Can you work these out from the model? Positions are in its coordinate system, mm. A direction names the side the tool comes from. Coordinates: 2 decimals unless noted, no trailing zeros. Loops run counter-clockwise (first coordinate to the right, second up) from the corner with the lowest first, then second, coordinate; pieces in that order, holes last. Notation, with made-up numbers: M 64.25,16 L 91.25,16 A33 ccw 91.25,49 Z; hole C 12.25,56.25 d9. An arc over 180 degrees is marked long. Answer as a JSON object with one key per item and string values. Group by question number.
Item 1: We'd pull the mould along Y, two halves only. Please class faces 1 (the cylindrical face through (8.374, 22.311, 0.369)), 2 (the cylindrical face through (-7.58, 9.664, -34.278)), 3 (the flat face through (-11, 38.1, 0)), 4 (the cylindrical face through (1.955, 8.803, -37.182)): +Y half, -Y half, draft (parallel to the pull), parting line (faces both ways), or undercut.
Item 2: Which directions (+Z, -Z, +X, -X, +Y, -Y) give clear straight access to the entire face, cutting with the end or side of a thin tool? Please do faces 5 (the cylindrical face through (6.65, 34.28, 9.5)), 6 (the cylindrical face through (11.356, 34.278, 0.473)), 7 (the cylindrical face through (-11.356, -0.473, -34.278)), 8 (the flat face through (7, -7, 30.48)), 9 (the cylindrical face through (-15.93, 5.02, 34.34)).
Item 3: Suppose I cut it at D-D (z = 27). Write out the boundary of the cut face in (x, y) (3 decimals).
Item 4: Suppose I cut it at B-B (y = 33). Write out the boundary of the cut face in (x, z), then the cut area to 3 significant figures.
Item 5: If I drill on line 1 (X direction, y = 34.5, z = 0); line 2 (Z direction, x = 12.5, y = -9); line 3 (Z direction, x = 0, y = 26) (3 decimals), over which ranges is the centre line in solid material (lowest first)?
Item 6: Suppose I cut it at A-A (z = 0). Count the separate pieces of the cut face and the enclosed holes in it, then the cut area to 3 significant figures.
Item 7: I'm going to push flat-ended pins straight in: pin 1 Ø4 at (x, z) = (1.5, -22.5) entering from +Y (3 decimals); pin 2 Ø4 at (y, z) = (31, 16) entering from -X; pin 3 Ø10 at (x, y) = (0, 0) entering from +Z; pin 4 Ø10 at (x, y) = (2, 32) entering from +Z. Where does each tip first touch, or does it pass through?
```python
from build123d import *

# Parameters (mm, degrees)
CIRPATTERN1_COUNT  = 6
CIRPATTERN5_COUNT  = 3
CIRPATTERN5_ANGLE  = 180
SKETCH6_R          = 8.382
CUT_EXTRUDE1_DEPTH = 50.8
SKETCH7_R          = 8.382
CUT_EXTRUDE2_DEPTH = 50.8


with BuildPart() as part:
    # Sketch3 → Revolve1 (revolve)
    with BuildSketch(Plane(origin=(0, 0, 0), x_dir=(0, 0, -1), z_dir=(1, 0, 0)), mode=Mode.PRIVATE) as revolve1_sk:
        Polygon((30.48, 9.525), (30.48, 16.7005), (38.1, 16.7005), (38.1, 10.795), (37.126090628, 10.795), (37.4396, 9.017), (36.9316, 9.017), (36.9316, 0), (0, 0), (0, 9.525), align=None)
    revolve1 = revolve(revolve1_sk.sketch.rotate(Axis((0, 0, -80.9), (0, 0, 1)), 90), axis=Axis((0, 0, -80.9), (0, 0, 1)))

    # Sketch4 → 11_64 _0.17188_ Diameter Hole1 (revolve, cut)
    with BuildSketch(Plane(origin=(-13.4874, 0, -38.1), x_dir=(0, 1, 0), z_dir=(1, 0, 0))):
        Polygon((0, 0), (0, 8.931604225), (2.182876, 7.62), (2.182876, 0.128524), (2.3114, 0), align=None)
    f_11_64_0_17188_diameter_hole1 = revolve(axis=Axis((-13.4874, 0, -44.45), (0, 0, 1)), mode=Mode.SUBTRACT)

    # CirPattern1: 11_64 _0.17188_ Diameter Hole1 ×6 about axis
    cirpattern1_axis = Axis((0, 0, 0), (0, 0, 1))
    for i in range(1, CIRPATTERN1_COUNT):
        add(f_11_64_0_17188_diameter_hole1.rotate(cirpattern1_axis, i * 360 / CIRPATTERN1_COUNT), mode=Mode.SUBTRACT)

    # CirPattern5: Revolve1, 11_64 _0.17188_ Diameter Hole1 ×3 about axis
    cirpattern5_axis = Axis((0, 0, 0), (1, 0, 0))
    add([revolve1.rotate(cirpattern5_axis, i * CIRPATTERN5_ANGLE / (CIRPATTERN5_COUNT - 1)) for i in range(1, CIRPATTERN5_COUNT)])
    add([f_11_64_0_17188_diameter_hole1.rotate(cirpattern5_axis, i * CIRPATTERN5_ANGLE / (CIRPATTERN5_COUNT - 1)) for i in range(1, CIRPATTERN5_COUNT)], mode=Mode.SUBTRACT)

    # CirPattern5 copy 1 sketch → CirPattern5 copy 1 (revolve, cut)
    with BuildSketch(Plane(origin=(-6.7437, 38.1, -11.680431031), x_dir=(-0.8660254037844386, -1.745740669421567e-15, 0.5000000000000001), z_dir=(0.5000000000000001, -3.023711536277457e-15, 0.8660254037844386))):
        Polygon((0, 0), (0, 8.931604225), (2.182876, 7.62), (2.182876, 0.128524), (2.3114, 0), align=None)
    revolve(axis=Axis((-6.7437, 44.45, -11.680431031), (0, -1, 0)), mode=Mode.SUBTRACT)

    # CirPattern5 copy 2 sketch → CirPattern5 copy 2 (revolve, cut)
    with BuildSketch(Plane(origin=(-6.7437, 11.680431031, 38.1), x_dir=(-0.8660254037844386, -0.5000000000000001, -3.491481338843134e-15), z_dir=(0.5000000000000001, -0.8660254037844386, -6.047423072554914e-15))):
        Polygon((0, 0), (0, 8.931604225), (2.182876, 7.62), (2.182876, 0.128524), (2.3114, 0), align=None)
    revolve(axis=Axis((-6.7437, 11.680431031, 44.45), (0, 0, -1)), mode=Mode.SUBTRACT)

    # CirPattern5 copy 3 sketch → CirPattern5 copy 3 (revolve, cut)
    with BuildSketch(Plane(origin=(6.7437, 38.1, -11.680431031), x_dir=(-0.8660254037844387, 1.7457406694215659e-15, -0.4999999999999998), z_dir=(-0.4999999999999998, -3.0237115362774574e-15, 0.8660254037844387))):
        Polygon((0, 0), (0, 8.931604225), (2.182876, 7.62), (2.182876, 0.128524), (2.3114, 0), align=None)
    revolve(axis=Axis((6.7437, 44.45, -11.680431031), (0, -1, 0)), mode=Mode.SUBTRACT)

    # CirPattern5 copy 4 sketch → CirPattern5 copy 4 (revolve, cut)
    with BuildSketch(Plane(origin=(6.7437, 11.680431031, 38.1), x_dir=(-0.8660254037844387, 0.4999999999999998, 3.4914813388431318e-15), z_dir=(-0.4999999999999998, -0.8660254037844387, -6.047423072554915e-15))):
        Polygon((0, 0), (0, 8.931604225), (2.182876, 7.62), (2.182876, 0.128524), (2.3114, 0), align=None)
    revolve(axis=Axis((6.7437, 11.680431031, 44.45), (0, 0, -1)), mode=Mode.SUBTRACT)

    # CirPattern5 copy 5 sketch → CirPattern5 copy 5 (revolve, cut)
    with BuildSketch(Plane(origin=(13.4874, 38.1, 0), x_dir=(0, 0, -1), z_dir=(-1, 0, 0))):
        Polygon((0, 0), (0, 8.931604225), (2.182876, 7.62), (2.182876, 0.128524), (2.3114, 0), align=None)
    revolve(axis=Axis((13.4874, 44.45, 0), (0, -1, 0)), mode=Mode.SUBTRACT)

    # CirPattern5 copy 6 sketch → CirPattern5 copy 6 (revolve, cut)
    with BuildSketch(Plane(origin=(13.4874, 0, 38.1), x_dir=(0, 1, 0), z_dir=(-1, 0, 0))):
        Polygon((0, 0), (0, 8.931604225), (2.182876, 7.62), (2.182876, 0.128524), (2.3114, 0), align=None)
    revolve(axis=Axis((13.4874, 0, 44.45), (0, 0, -1)), mode=Mode.SUBTRACT)

    # CirPattern5 copy 7 sketch → CirPattern5 copy 7 (revolve, cut)
    with BuildSketch(Plane(origin=(6.7437, 38.1, 11.680431031), x_dir=(0.8660254037844384, 1.7457406694215683e-15, -0.5000000000000004), z_dir=(-0.5000000000000004, 3.0237115362774562e-15, -0.8660254037844384))):
        Polygon((0, 0), (0, 8.931604225), (2.182876, 7.62), (2.182876, 0.128524), (2.3114, 0), align=None)
    revolve(axis=Axis((6.7437, 44.45, 11.680431031), (0, -1, 0)), mode=Mode.SUBTRACT)

    # CirPattern5 copy 8 sketch → CirPattern5 copy 8 (revolve, cut)
    with BuildSketch(Plane(origin=(6.7437, -11.680431031, 38.1), x_dir=(0.8660254037844384, 0.5000000000000004, 3.4914813388431365e-15), z_dir=(-0.5000000000000004, 0.8660254037844384, 6.0474230725549124e-15))):
        Polygon((0, 0), (0, 8.931604225), (2.182876, 7.62), (2.182876, 0.128524), (2.3114, 0), align=None)
    revolve(axis=Axis((6.7437, -11.680431031, 44.45), (0, 0, -1)), mode=Mode.SUBTRACT)

    # CirPattern5 copy 9 sketch → CirPattern5 copy 9 (revolve, cut)
    with BuildSketch(Plane(origin=(-6.7437, 38.1, 11.680431031), x_dir=(0.8660254037844386, -1.745740669421567e-15, 0.5000000000000001), z_dir=(0.5000000000000001, 3.023711536277457e-15, -0.8660254037844386))):
        Polygon((0, 0), (0, 8.931604225), (2.182876, 7.62), (2.182876, 0.128524), (2.3114, 0), align=None)
    revolve(axis=Axis((-6.7437, 44.45, 11.680431031), (0, -1, 0)), mode=Mode.SUBTRACT)

    # CirPattern5 copy 10 sketch → CirPattern5 copy 10 (revolve, cut)
    with BuildSketch(Plane(origin=(-6.7437, -11.680431031, 38.1), x_dir=(0.8660254037844386, -0.5000000000000001, -3.491481338843134e-15), z_dir=(0.5000000000000001, 0.8660254037844386, 6.047423072554914e-15))):
        Polygon((0, 0), (0, 8.931604225), (2.182876, 7.62), (2.182876, 0.128524), (2.3114, 0), align=None)
    revolve(axis=Axis((-6.7437, -11.680431031, 44.45), (0, 0, -1)), mode=Mode.SUBTRACT)

    # Sketch6 → Cut-Extrude1 (cut, symmetric)
    with BuildSketch(Plane.XY):
        with Locations(Location((0, 0, 0), (0, 0, 270))):
            Circle(SKETCH6_R)
    extrude(amount=CUT_EXTRUDE1_DEPTH, both=True, mode=Mode.SUBTRACT)

    # Sketch7 → Cut-Extrude2 (cut)
    with BuildSketch(Plane(origin=(0, 0, 0), x_dir=(1, 0, 0), z_dir=(0, 1, 0))):
        with Locations(Location((0, 0, 0), (0, 0, 180))):
            Circle(SKETCH7_R)
    extrude(amount=CUT_EXTRUDE2_DEPTH, mode=Mode.SUBTRACT)


solid = part.part
```
From the geometry:
{
 "1": {"face 1": "draft", "face 2": "undercut", "face 3": "+Y half", "face 4": "undercut"},
 "2": {"face 5": "+Y", "face 6": "+Y, -Y", "face 7": "+Z, -Z", "face 8": "none", "face 9": "+Z"},
 "3": {"outline": "C 0,0 d19.05; hole C 0,0 d16.764"},
 "4": {"outline": "C 0,0 d33.4; hole C -13.49,0 d4.37; hole C -6.74,-11.68 d4.37; hole C -6.74,11.68 d4.37; hole C 0,0 d16.76; hole C 6.74,-11.68 d4.37; hole C 6.74,11.68 d4.37; hole C 13.49,0 d4.37", "area": "566 mm2"},
 "5": {"line 1": "-16.7 to -15.67, -11.3 to -8.38, 8.38 to 11.3, 15.67 to 16.7", "line 2": "-38.1 to -30.48, 30.48 to 38.1", "line 3": "-9.525 to -8.382, 8.382 to 9.525"},
 "6": {"separate pieces": "3", "enclosed holes": "0", "area": "158 mm2"},
 "7": {"pin 1": "y = 9.525", "pin 2": "x = -9.11", "pin 3": "through", "pin 4": "z = 16.7"}
}
